For this review, take the finished solid that the model builds, in its own axes (mm). Face numbers are marked on the shaded views. A direction names the side the tool comes from. Round coordinates to 2 decimals unless told otherwise and drop trailing zeros. Write each loop counter-clockwise with the first axis right and the second up, starting at its lowest first coordinate (ties: lowest second). Pieces come first, ordered by that corner, then holes. Notation, with made-up numbers: (67, 14) -> (75, 14) arc R26 ccw to (75, 46) -> close; hole circle Ø7 at (-6.75, 74.5). An arc over 180 degrees is marked (long way). Answer as CSV lines item,"result". Start each with the question number.
Item 1: Machinability: for the marked faces 5 and 6, which of the approach directions +Z, -Z, +X, -X, +Y, -Y give a long, thin tool a straight path to every point of the face, cutting with its end or side? Answer none if there is none.
Item 2: Mouldability with a two-part tool opening along X and no side actions: class the marked faces 1, 2, 3 and 4 as +X half, -X half, draft (parallel to the pull), parting line (faces both ways), or undercut.
Item 3: Take a section at B-B on y = -1. Give the boundary of the cut face in (x, z), then the cut area to 3 significant figures.
Item 4: Wall thickness on probe 1 along X at (y, z) = (-17.5, -3.5); probe 2 along Z at (x, y) = (-17, 9); probe 3 along Z at (x, y) = (-13.5, -19): over which ranges is each line inside the solid? List them lowest first. Write a range as from..to.
Item 5: Take a section at D-D on x = 0. Give the boundary of the cut face in (y, z), then the cut area to 3 significant figures.
Item 6: Take a section at A-A on x = 33. Give the boundary of the cut face in (y, z).
Item 7: For pin 1 Ø1 at (x, y) = (21.5, -11.5) entering from +Z; pin 2 Ø1.3 at (y, z) = (7, -13) entering from -X; pin 3 Ø6 at (x, y) = (21, 13.5) entering from -Z, all flat-tipped, find the tip position at first contact; note any pin that passes through.
Item 8: Take a section at C-C on z = 8. Give the boundary of the cut face in (x, y), then the cut area to 3 significant figures.
```python
from build123d import *

# Parameters (mm, degrees)
F1_DEPTH = 25.4
F2_DEPTH = 12.7
F3_SIZE  = 5.08
F4_R     = 8.5094
F4_R_2   = 7.830617
F5_DEPTH = 29.464


with BuildPart() as f1:
    # F0 (on Front) → F1 (new body, symmetric)
    with BuildSketch(Plane.XZ):
        with BuildLine():
            Line((-28.034671, -4.311011), (-28.034671, -14.077194))
            Line((-28.034671, -14.077194), (27.299206, -14.022477))
            Line((27.299206, -14.022477), (27.299206, -7.378203))
            ThreePointArc((27.299206, -7.378203), (34.129328, -0.548081), (40.95945, -7.378203))
            Line((40.95945, -7.378203), (40.95945, -14.022477))
            Line((40.95945, -14.022477), (55.595427, -14.055348))
            Line((55.595427, -14.055348), (55.595427, -8.005464))
            Line((55.595427, -8.005464), (49.564611, -8.005464))
            Line((49.564611, -8.005464), (49.564611, 3.545878))
            Line((49.564611, 3.545878), (20.311819, 3.713833))
            Line((20.311819, 3.713833), (20.311819, -7.577809))
            Line((20.311819, -7.577809), (-17.788181, -7.57786))
            Line((-17.788181, -7.57786), (-17.788197, 3.932584))
            Line((-17.788197, 3.932584), (-25.274342, 3.975565))
            Line((-25.274342, 3.975565), (-25.274342, 6.474282))
            Line((-25.274342, 6.474282), (-25.274342, 17.366793))
            Line((-25.274342, 17.366793), (-47.289753, 17.366793))
            Line((-47.289753, 17.366793), (-47.289753, 14.9899))
            Line((-47.289753, 14.9899), (-43.719519, 13.406432))
            Line((-43.719519, 13.406432), (-43.719519, -6.054001))
            Line((-43.719519, -6.054001), (-40.48594, -6.054001))
            Line((-40.48594, -6.054001), (-40.48594, -4.311011))
            ThreePointArc((-40.48594, -4.311011), (-34.260305, 1.219482), (-28.034671, -4.311011))
        make_face()
    extrude(amount=F1_DEPTH, both=True)

    # F0 (on Front) → F2 (join, symmetric)
    with BuildSketch(Plane.XZ):
        Polygon((20.311819, -7.577809), (20.311819, 3.713833), (1.920144, 3.819428), (-16.471527, 3.925024), (-17.788197, 3.932584), (-17.788181, -7.57786), align=None)
        with BuildLine():
            Line((-16.471527, 3.925024), (1.920144, 3.819428))
            Line((1.920144, 3.819428), (1.920144, 10.733619))
            ThreePointArc((1.920144, 10.733619), (-7.524811, 9.64175), (-16.47153, 6.42374))
            Line((-16.47153, 6.42374), (-16.471527, 3.925024))
        make_face()
        Polygon((-16.47153, 6.42374), (-25.274342, 6.474282), (-25.274342, 3.975565), (-17.788197, 3.932584), (-16.471527, 3.925024), align=None)
        with BuildLine():
            Line((1.920144, 3.819428), (20.311819, 3.713833))
            Line((20.311819, 3.713833), (20.311819, 6.42374))
            ThreePointArc((20.311819, 6.42374), (11.3651, 9.64175), (1.920144, 10.733619))
            Line((1.920144, 10.733619), (1.920144, 3.819428))
        make_face()
        Polygon((20.311819, 6.42374), (20.311819, 3.713833), (23.388268, 3.713833), (23.387096, 4.89868), align=None)
    extrude(amount=F2_DEPTH, both=True)

    # F3
    f3_edges = [f1.edges().sort_by_distance(p)[0] for p in [
        (49.564611, 25.4, -2.229793),
        (55.595427, 25.4, -11.030406),
        (49.564611, -25.4, -2.229793),
        (55.595427, -25.4, -11.030406),
    ]]
    chamfer(f3_edges, length=F3_SIZE)

    # F4 (on Front) → F5 (join, symmetric)
    with BuildSketch(Plane.XZ):
        with Locations((-33.875754, -7.361865)):
            Circle(F4_R)
        with Locations((33.989035, -8.773327)):
            Circle(F4_R_2)
    extrude(amount=F5_DEPTH, both=True)


solid = f1.part
```
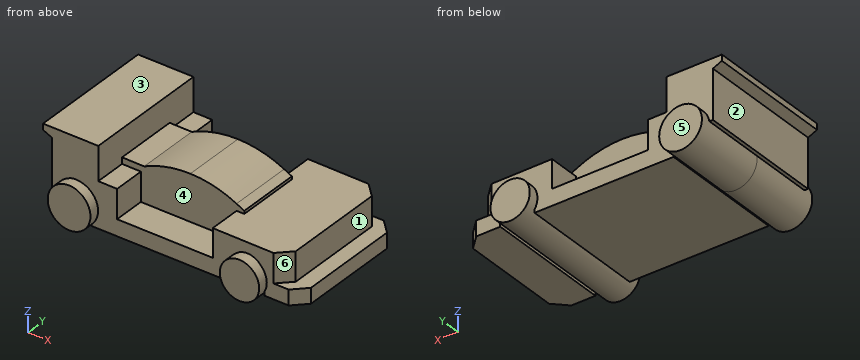
Output values:
1,face 5,"+Z, -Z, +X, -X, +Y"
1,face 6,"+Z, +X, -Y"
2,face 1,"+X half"
2,face 2,"-X half"
2,face 3,"draft"
2,face 4,"undercut"
3,outline,"(-47.29, 14.99) -> (-43.72, 13.41) -> (-43.72, -6.05) -> (-42.28, -6.05) arc R8.51 ccw to (-28.03, -13.55) -> (-28.03, -14.08) -> (27.3, -14.02) -> (27.3, -12.84) arc R7.83 ccw to (40.96, -12.34) -> (40.96, -14.02) -> (55.6, -14.06) -> (55.6, -8.01) -> (49.56, -8.01) -> (49.56, 3.55) -> (20.31, 3.71) -> (23.39, 3.71) -> (23.39, 4.9) -> (20.31, 6.42) arc R41.4 ccw to (1.92, 10.73) arc R41.4 ccw to (-16.47, 6.42) -> (-25.27, 6.47) -> (-25.27, 17.37) -> (-47.29, 17.37) -> close; hole (-37.34, 0.41) arc R8.51 cw to (-33.11, 1.11) arc R6.27 ccw to start; hole (29.5, -2.36) arc R7.83 cw to (39.67, -3.38) arc R6.83 ccw to start"
3,area,"2,200 mm^2"
4,probe 1,"x = -43.72..-17.79, 20.31..49.56"
4,probe 2,"z = -14.07..6.43"
4,probe 3,"z = -14.06..-7.58"
5,outline,"(-25.4, -14.05) -> (25.4, -14.05) -> (25.4, -7.58) -> (12.7, -7.58) -> (12.7, 10.69) -> (-12.7, 10.69) -> (-12.7, -7.58) -> (-25.4, -7.58) -> close"
5,area,"793 mm^2"
6,outline,"(-29.46, -16.54) -> (29.46, -16.54) -> (29.46, -1.01) -> (-29.46, -1.01) -> close; (-25.4, -0.64) -> (25.4, -0.64) -> (25.4, 3.64) -> (-25.4, 3.64) -> close"
7,pin 1,"stops at z = 6.08"
7,pin 2,"stops at x = -40.77"
7,pin 3,"stops at z = -14.03"
8,outline,"(-43.72, -25.4) -> (-25.27, -25.4) -> (-25.27, 25.4) -> (-43.72, 25.4) -> close; (-12.87, -12.7) -> (16.71, -12.7) -> (16.71, 12.7) -> (-12.87, 12.7) -> close"
8,area,"1,690 mm^2"
